from build123d import *

# Parameters (mm, degrees)
SKETCH_1_R      = 42.5
SKETCH_1_R_2    = 10
SKETCH_1_R_3    = 2.1
SKETCH_1_R_4    = 1.6
EXTRUDE_1_DEPTH = 5
FILLET_1_R      = 3


with BuildPart() as part:
    # 草图1 → 凸台-拉伸1 (new body)
    with BuildSketch(Plane(origin=(0, 0, 0), x_dir=(1, 0, 0), z_dir=(0, 1, 0))):
        with Locations(Location((0, 0, 0), (0, 0, 270))):
            Circle(SKETCH_1_R)
        with Locations(Location((0, 0, 0), (0, 0, 270))):
            Circle(SKETCH_1_R_2, mode=Mode.SUBTRACT)
        with Locations(Location((0, 14, 0), (0, 0, 270))):
            Circle(SKETCH_1_R_3, mode=Mode.SUBTRACT)
        with Locations(Location((12.124355653, 7, 0), (0, 0, 270))):
            Circle(SKETCH_1_R_3, mode=Mode.SUBTRACT)
        with Locations(Location((12.124355653, -7, 0), (0, 0, 270))):
            Circle(SKETCH_1_R_3, mode=Mode.SUBTRACT)
        with Locations(Location((0, -14, 0), (0, 0, 270))):
            Circle(SKETCH_1_R_3, mode=Mode.SUBTRACT)
        with Locations(Location((-12.124355653, -7, 0), (0, 0, 270))):
            Circle(SKETCH_1_R_3, mode=Mode.SUBTRACT)
        with Locations(Location((-12.124355653, 7, 0), (0, 0, 270))):
            Circle(SKETCH_1_R_3, mode=Mode.SUBTRACT)
        with Locations(Location((0, 38.5, 0), (0, 0, 270))):
            Circle(SKETCH_1_R_4, mode=Mode.SUBTRACT)
        with Locations(Location((19.25, 33.341978046, 0), (0, 0, 270))):
            Circle(SKETCH_1_R_4, mode=Mode.SUBTRACT)
        with Locations(Location((33.341978046, 19.25, 0), (0, 0, 270))):
            Circle(SKETCH_1_R_4, mode=Mode.SUBTRACT)
        with Locations(Location((38.5, 0, 0), (0, 0, 270))):
            Circle(SKETCH_1_R_4, mode=Mode.SUBTRACT)
        with Locations(Location((33.341978046, -19.25, 0), (0, 0, 270))):
            Circle(SKETCH_1_R_4, mode=Mode.SUBTRACT)
        with Locations(Location((19.25, -33.341978046, 0), (0, 0, 270))):
            Circle(SKETCH_1_R_4, mode=Mode.SUBTRACT)
        with Locations(Location((0, -38.5, 0), (0, 0, 270))):
            Circle(SKETCH_1_R_4, mode=Mode.SUBTRACT)
        with Locations(Location((-19.25, -33.341978046, 0), (0, 0, 270))):
            Circle(SKETCH_1_R_4, mode=Mode.SUBTRACT)
        with Locations(Location((-33.341978046, -19.25, 0), (0, 0, 270))):
            Circle(SKETCH_1_R_4, mode=Mode.SUBTRACT)
        with Locations(Location((-38.5, 0, 0), (0, 0, 270))):
            Circle(SKETCH_1_R_4, mode=Mode.SUBTRACT)
        with Locations(Location((-33.341978046, 19.25, 0), (0, 0, 270))):
            Circle(SKETCH_1_R_4, mode=Mode.SUBTRACT)
        with Locations(Location((-19.25, 33.341978046, 0), (0, 0, 270))):
            Circle(SKETCH_1_R_4, mode=Mode.SUBTRACT)
        with Locations(Location((-27.279800219, 15.75, 0), (0, 0, 270))):
            Circle(SKETCH_1_R_4, mode=Mode.SUBTRACT)
        with Locations(Location((-21.217622393, 12.25, 0), (0, 0, 270))):
            Circle(SKETCH_1_R_4, mode=Mode.SUBTRACT)
        with Locations(Location((-17.320508076, 10, 0), (0, 0, 270))):
            Circle(SKETCH_1_R_4, mode=Mode.SUBTRACT)
        with Locations(Location((27.279800219, 15.75, 0), (0, 0, 270))):
            Circle(SKETCH_1_R_4, mode=Mode.SUBTRACT)
        with Locations(Location((21.217622393, 12.25, 0), (0, 0, 270))):
            Circle(SKETCH_1_R_4, mode=Mode.SUBTRACT)
        with Locations(Location((17.320508076, 10, 0), (0, 0, 270))):
            Circle(SKETCH_1_R_4, mode=Mode.SUBTRACT)
        with Locations(Location((0, -31.5, 0), (0, 0, 270))):
            Circle(SKETCH_1_R_4, mode=Mode.SUBTRACT)
        with Locations(Location((0, -24.5, 0), (0, 0, 270))):
            Circle(SKETCH_1_R_4, mode=Mode.SUBTRACT)
        with Locations(Location((0, -20, 0), (0, 0, 270))):
            Circle(SKETCH_1_R_4, mode=Mode.SUBTRACT)
        with BuildLine():
            Line((-25, 24.494897428), (-14.285714286, 13.997084244))
            ThreePointArc((-14.285714286, 13.997084244), (0, 20), (14.285714286, 13.997084244))
            Line((14.285714286, 13.997084244), (25, 24.494897428))
            ThreePointArc((25, 24.494897428), (0, 35), (-25, 24.494897428))
        make_face(mode=Mode.SUBTRACT)
        with BuildLine():
            Line((8.713203436, -33.898083809), (4.978973392, -19.370333605))
            ThreePointArc((4.978973392, -19.370333605), (17.320508076, -10), (19.264687677, 5.37324936))
            Line((19.264687677, 5.37324936), (33.713203436, 9.403186381))
            ThreePointArc((33.713203436, 9.403186381), (30.310889132, -17.5), (8.713203436, -33.898083809))
        make_face(mode=Mode.SUBTRACT)
        with BuildLine():
            Line((-33.713203436, 9.403186381), (-19.264687677, 5.37324936))
            ThreePointArc((-19.264687677, 5.37324936), (-17.320508076, -10), (-4.978973392, -19.370333605))
            Line((-4.978973392, -19.370333605), (-8.713203436, -33.898083809))
            ThreePointArc((-8.713203436, -33.898083809), (-30.310889132, -17.5), (-33.713203436, 9.403186381))
        make_face(mode=Mode.SUBTRACT)
    extrude(amount=EXTRUDE_1_DEPTH)

    # 圆角1
    fillet_1_edges = [part.edges().sort_by_distance(p)[0] for p in [
        (8.713203436, 2.5, 33.898083809),
        (33.713203436, 2.5, -9.403186381),
        (19.264687677, 2.5, -5.37324936),
        (4.978973392, 2.5, 19.370333605),
        (-33.713203436, 2.5, -9.403186381),
        (-8.713203436, 2.5, 33.898083809),
        (-4.978973392, 2.5, 19.370333605),
        (-19.264687677, 2.5, -5.37324936),
        (25, 2.5, -24.494897428),
        (-25, 2.5, -24.494897428),
        (-14.285714286, 2.5, -13.997084244),
        (14.285714286, 2.5, -13.997084244),
    ]]
    fillet(fillet_1_edges, radius=FILLET_1_R)


solid = part.part
The listing builds one solid part. Answer for the finished solid, in the listing's coordinates (mm). Coordinates: 2 decimals unless noted, no trailing zeros. Write each loop counter-clockwise with the first axis right and the second up, starting at its lowest first coordinate (ties: lowest second). Pieces come first, ordered by that corner, then holes. Notation, with made-up numbers: (51.25, 10) - (88.25, 10) arc R35 cw to (88.25, 43) - close; hole circle Ø10 at (54, 11). An arc over 180 degrees is marked (long way). Answer as CSV lines item,"result".
1. Determine the mould class of faces 1 (the flat face through (-9, 0, 9)), 2 (the cylindrical face through (1.08, 2.46, 23.32)), 3 (the cylindrical face through (-25.861, 2.465, -33.727)) for opening direction Z: +Z half, -Z half, draft (parallel to the pull), parting line (faces both ways), or undercut.
Computed values:
face 1,"draft"
face 2,"undercut"
face 3,"parting line"
2. Find section B-B (x = -4). Give the vertices of the cut face in (y, z).
Computed values:
outline,"(0, -42.31) - (5, -42.31) - (5, -34.77) - (0, -34.77) - close; (0, -19.6) - (5, -19.6) - (5, -9.17) - (0, -9.17) - close; (0, 9.17) - (5, 9.17) - (5, 42.31) - (0, 42.31) - close"
3. Given P1, Ø3, axis at y = 1.5, z = -1.5, coming from the +X side; P2, Ø3, axis at x = -21.22, z = -12.25, coming from the -Y side; P3, Ø3, axis at x = 27.5, y = 2, coming from the -Z side, each flat-ended and moving along its own axis, determine where each tip first touches the part or whether it passes through.
Computed values:
P1,"stops at x = 42.5"
P2,"passes through"
P3,"stops at z = -33.62"
4. Find section D-D (y = 2.95). Give the number of separate pieces and of enclosed holes in the cut face, plus the area to 3 significant figures.
Computed values:
separate pieces,"1"
enclosed holes,"31"
area,"3,160 mm²"
5. Find section C-C (z = 3.5). Give the vertices of the cut face in (x, y), plus the area to 3 significant figures.
Computed values:
outline,"(-42.36, 0) - (-34.82, 0) - (-34.82, 5) - (-42.36, 5) - close; (-19.69, 0) - (-9.37, 0) - (-9.37, 5) - (-19.69, 5) - close; (9.37, 0) - (19.69, 0) - (19.69, 5) - (9.37, 5) - close; (34.82, 0) - (42.36, 0) - (42.36, 5) - (34.82, 5) - close"
area,"179 mm²"
6. Straight lines are drawn through the part: line 1 (Z direction, x = -9, y = 4.5); line 2 (X direction, y = 1.45, z = 15.5); line 3 (Z direction, x = 5, y = 1.15). For each, find the intervals that lie inside material, in ascending order. Write a range as [from, to].
Computed values:
line 1,"z = [-41.54, -33.82], [-17.86, -4.36], [4.36, 17.86], [32.48, 41.54]"
line 2,"x = [-39.57, -31.38], [-12.64, -1.47], [1.47, 12.64], [31.38, 39.57]"
line 3,"z = [-42.2, -34.64], [-19.36, -8.66], [8.66, 42.2]"
7. Find section A-A (z = 38.5). Give the vertices of the cut face in (x, y), plus the area to 3 significant figures.
Computed values:
outline,"(-18, 0) - (-1.6, 0) - (-1.6, 5) - (-18, 5) - close; (1.6, 0) - (18, 0) - (18, 5) - (1.6, 5) - close"
area,"164 mm²"
